Job drawing, mm, ordinate dimensions from the low corner. One solid piece. Round coordinates to 2 decimals unless told otherwise and drop trailing zeros. Order: outer loops, then holes, each group sorted by start corner. A loop starts at its lowest first (then second) coordinate and runs counter-clockwise, first axis right, second up. Notation, with made-up numbers: (61, -38) -> (98, -38) arc R19 cw to (98, -1) -> close; hole circle Ø6 at (-29, 29.25). An arc over 180 degrees is marked (long way). Write item = value, one per line.
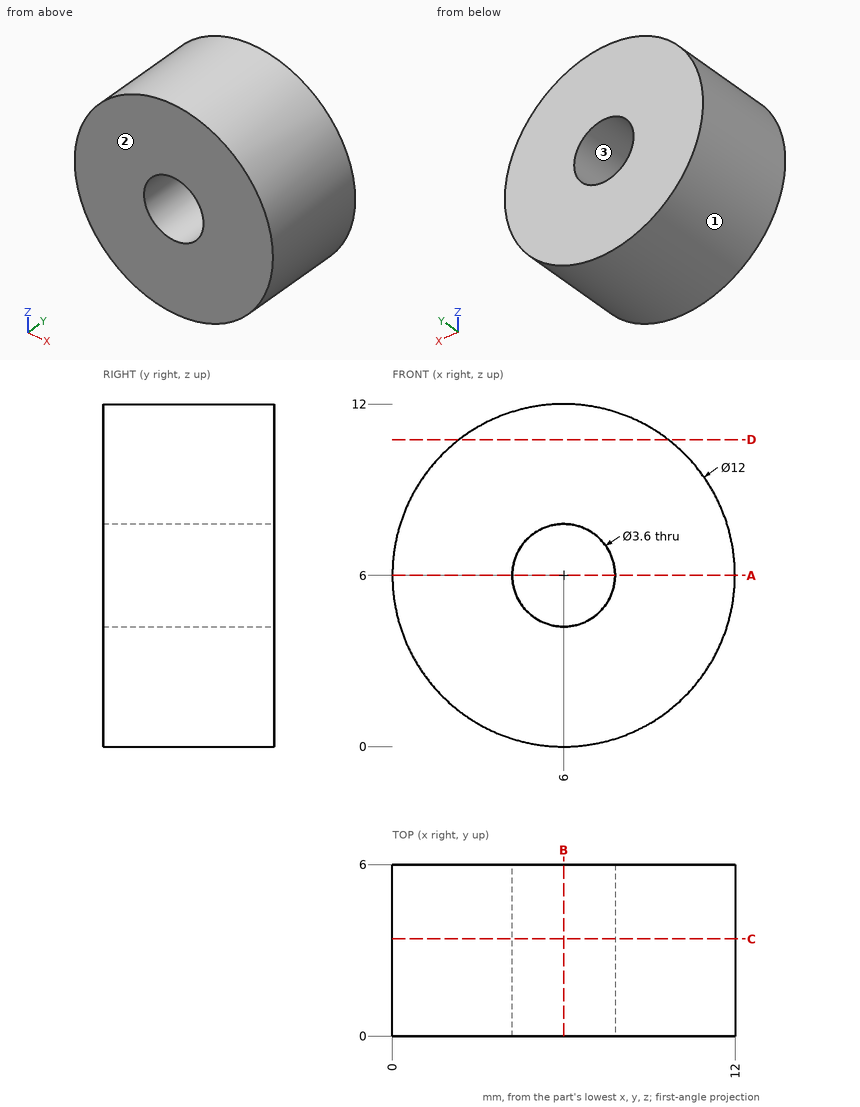
Q1. Cut at B-B, the plane x = 6. List the corners of the cut face in (y, z), and give its area (3 significant figures).
Check values:
outline = (0, 0) -> (6, 0) -> (6, 4.2) -> (0, 4.2) -> close; (0, 7.8) -> (6, 7.8) -> (6, 12) -> (0, 12) -> close
area = 50.4 mm²
Q2. Probe probe 1 along Z at (x, y) = (6, 2.2); probe 2 along X at (y, z) = (3.85, 5.75); probe 3 along Z at (x, y) = (7.5, 1.35). List the from-to ranges inside material, lowest first.
Check values:
probe_1 = 0 to 4.2, 7.8 to 12
probe_2 = 0.01 to 4.22, 7.78 to 11.99
probe_3 = 0.19 to 5.01, 6.99 to 11.81
Q3. Mould opens along Z. For the marked faces 1, 2 and 3 say: released by +Z, released by -Z, zero draft, split by the parting line, or undercut.
Check values:
face_1 = split by the parting line
face_2 = zero draft
face_3 = undercut
Q4. Cut at D-D, the plane z = 10.75. List the corners of the cut face in (x, y).
Check values:
outline = (2.33, 0) -> (9.67, 0) -> (9.67, 6) -> (2.33, 6) -> close
Q5. Cut at C-C, the plane y = 3.4. List the corners of the cut face in (x, z), and give its area (3 significant figures).
Check values:
outline = circle Ø12 at (6, 6); hole circle Ø3.6 at (6, 6)
area = 103 mm²
Q6. Cut at A-A, the plane z = 6. List the corners of the cut face in (x, y), and give its area (3 significant figures).
Check values:
outline = (0, 0) -> (4.2, 0) -> (4.2, 6) -> (0, 6) -> close; (7.8, 0) -> (12, 0) -> (12, 6) -> (7.8, 6) -> close
area = 50.4 mm²
Q7. Flat gauge pins, fed straight in: pin 1 (2 mm diameter, centred on y = 2, z = 2.5, fed in from +X); pin 2 (3 mm diameter, centred on x = 10.5, y = 3.5, fed in from +Z). Where does each tip first touch, or does it go through?
Check values:
pin_1 = 11.45
pin_2 = 11.2
